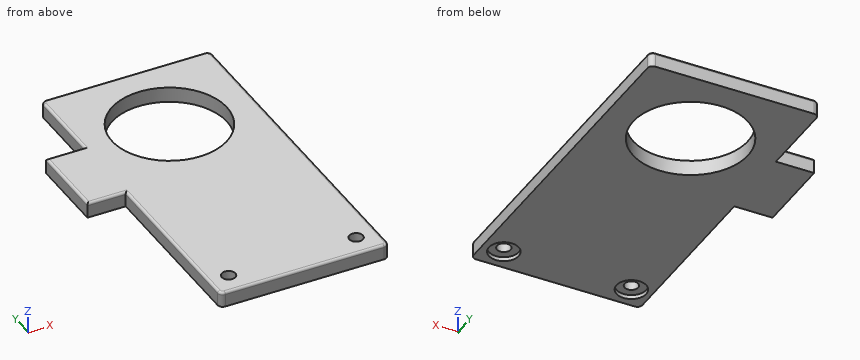
from build123d import *

# Parameters (mm, degrees)
SKETCH_1_R          = 6.75
EXTRUDE_1_DEPTH     = 1.8
SKETCH_2_R          = 0.8
CUT_EXTRUDE_1_DEPTH = 2
SKETCH_3_R          = 1.75
CUT_EXTRUDE_2_DEPTH = 0.5
SKETCH_4_W          = 4.5
SKETCH_4_H          = 9.8
EXTRUDE_2_DEPTH     = 1.8
SKETCH_5_R          = 1.75
EXTRUDE_3_DEPTH     = 1.3
SKETCH_6_R          = 1.75
EXTRUDE_4_DEPTH     = 1.8
EXTRUDE_5_DEPTH     = 1.8
CUT_EXTRUDE_3_DEPTH = 10
FILLET_1_R          = 0.7
CUT_EXTRUDE_4_DEPTH = 10
FILLET_2_R          = 0.3


with BuildPart() as part:
    # 草图1 → 凸台-拉伸1 (new body)
    with BuildSketch(Plane.XY):
        with BuildLine():
            Line((0.7, 0), (19.5, 0))
            ThreePointArc((19.5, 0), (19.994974747, -0.205025253), (20.2, -0.7))
            Line((20.2, -0.7), (20.2, -39.6))
            ThreePointArc((20.2, -39.6), (19.994974747, -40.094974747), (19.5, -40.3))
            Line((19.5, -40.3), (0.7, -40.3))
            ThreePointArc((0.7, -40.3), (0.205025253, -40.094974747), (0, -39.6))
            Line((0, -39.6), (0, -0.7))
            ThreePointArc((0, -0.7), (0.205025253, -0.205025253), (0.7, 0))
        make_face()
        with Locations((10.1, -10.1)):
            Circle(SKETCH_1_R, mode=Mode.SUBTRACT)
    extrude(amount=EXTRUDE_1_DEPTH)

    # 草图2 → 切除-拉伸1 (cut)
    with BuildSketch(Plane.XY.offset(1.8)):
        with Locations((17.6, -2.6)):
            Circle(SKETCH_2_R)
        with Locations((17.6, -37.6)):
            Circle(SKETCH_2_R)
        with Locations((2.6, -37.6)):
            Circle(SKETCH_2_R)
        with Locations((2.6, -2.6)):
            Circle(SKETCH_2_R)
    extrude(amount=-CUT_EXTRUDE_1_DEPTH, mode=Mode.SUBTRACT)

    # 草图3 → 切除-拉伸2 (cut)
    with BuildSketch(Plane(origin=(0, 0, 0), x_dir=(-1, 0, 0), z_dir=(0, 0, -1))):
        with Locations((-17.6, -2.6)):
            Circle(SKETCH_3_R)
        with Locations((-2.6, -2.6)):
            Circle(SKETCH_3_R)
        with Locations((-17.6, -37.6)):
            Circle(SKETCH_3_R)
        with Locations((-2.6, -37.6)):
            Circle(SKETCH_3_R)
    extrude(amount=-CUT_EXTRUDE_2_DEPTH, mode=Mode.SUBTRACT)

    # 草图4 → 凸台-拉伸2 (add)
    with BuildSketch(Plane(origin=(0, 0, 0), x_dir=(-1, 0, 0), z_dir=(0, 0, -1))):
        with Locations((2.25, -14.4)):
            Rectangle(SKETCH_4_W, SKETCH_4_H)
    extrude(amount=-EXTRUDE_2_DEPTH)

    # 草图5 → 凸台-拉伸3 (add)
    with BuildSketch(Plane(origin=(0, 0, 0.5), x_dir=(-1, 0, 0), z_dir=(0, 0, -1))):
        with Locations((-2.6, -2.6)):
            Circle(SKETCH_5_R)
        with Locations((-17.6, -2.6)):
            Circle(SKETCH_5_R)
    extrude(amount=-EXTRUDE_3_DEPTH)

    # 草图6 → 凸台-拉伸4 (add)
    with BuildSketch(Plane(origin=(0, 0, 0), x_dir=(-1, 0, 0), z_dir=(0, 0, -1))):
        with Locations((-17.6, -2.6)):
            Circle(SKETCH_6_R)
        with Locations((-2.6, -2.6)):
            Circle(SKETCH_6_R)
    extrude(amount=-EXTRUDE_4_DEPTH)

    # 草图8 → 凸台-拉伸5 (add)
    with BuildSketch(Plane(origin=(0, 0, 0), x_dir=(-1, 0, 0), z_dir=(0, 0, -1))):
        Polygon((-0.7, 0), (0, 0), (0, -0.7), align=None)
        Polygon((-0.7, -40.3), (0, -40.3), (0, -39.6), align=None)
    extrude(amount=-EXTRUDE_5_DEPTH)

    # 草图9 → 切除-拉伸3 (cut)
    with BuildSketch(Plane(origin=(0, 0, 0), x_dir=(-1, 0, 0), z_dir=(0, 0, -1))):
        Polygon((0, -19.3), (0, -40.3), (-0.15, -40.3), (-0.15, -19.15), (4.35, -19.15), (4.35, -9.65), (-0.15, -9.65), (-0.15, 0), (0, 0), (0, -9.5), (4.5, -9.5), (4.5, -19.3), align=None)
    extrude(amount=-CUT_EXTRUDE_3_DEPTH, mode=Mode.SUBTRACT)

    # 圆角1
    fillet_1_edges = [part.edges().sort_by_distance(p)[0] for p in [
        (0.15, -40.3, 0.9),
        (0.15, 0, 0.9),
    ]]
    fillet(fillet_1_edges, radius=FILLET_1_R)

    # 草图10 → 切除-拉伸4 (cut)
    with BuildSketch(Plane(origin=(0, 0, 0), x_dir=(-1, 0, 0), z_dir=(0, 0, -1))):
        with BuildLine():
            ThreePointArc((-20.2, -39.6), (-19.994974747, -40.094974747), (-19.5, -40.3))
            Line((-19.5, -40.3), (-0.85, -40.3))
            ThreePointArc((-0.85, -40.3), (-0.355025253, -40.094974747), (-0.15, -39.6))
            Line((-0.15, -39.6), (-0.15, -19.15))
            Line((-0.15, -19.15), (4.35, -19.15))
            Line((4.35, -19.15), (4.35, -9.65))
            Line((4.35, -9.65), (-0.15, -9.65))
            Line((-0.15, -9.65), (-0.15, -0.7))
            ThreePointArc((-0.15, -0.7), (-0.355025253, -0.205025253), (-0.85, 0))
            Line((-0.85, 0), (-19.5, 0))
            ThreePointArc((-19.5, 0), (-19.994974747, -0.205025253), (-20.2, -0.7))
            Line((-20.2, -0.7), (-20.2, -39.6))
        make_face()
        with BuildLine():
            ThreePointArc((-20.1, -39.6), (-19.924264069, -40.024264069), (-19.5, -40.2))
            Line((-19.5, -40.2), (-0.85, -40.2))
            ThreePointArc((-0.85, -40.2), (-0.425735931, -40.024264069), (-0.25, -39.6))
            Line((-0.25, -39.6), (-0.25, -19.05))
            Line((-0.25, -19.05), (4.25, -19.05))
            Line((4.25, -19.05), (4.25, -9.75))
            Line((4.25, -9.75), (-0.25, -9.75))
            Line((-0.25, -9.75), (-0.25, -0.7))
            ThreePointArc((-0.25, -0.7), (-0.425735931, -0.275735931), (-0.85, -0.1))
            Line((-0.85, -0.1), (-19.5, -0.1))
            ThreePointArc((-19.5, -0.1), (-19.924264069, -0.275735931), (-20.1, -0.7))
            Line((-20.1, -0.7), (-20.1, -39.6))
        make_face(mode=Mode.SUBTRACT)
    extrude(amount=-CUT_EXTRUDE_4_DEPTH, mode=Mode.SUBTRACT)

    # 圆角2
    fillet_2_edges = [part.edges().sort_by_distance(p)[0] for p in [
        (19.924264069, -40.024264069, 1.8),
        (10.175, -40.2, 1.8),
        (0.425735931, -40.024264069, 1.8),
        (0.25, -29.325, 1.8),
        (-2, -19.05, 1.8),
        (-4.25, -14.4, 1.8),
        (-2, -9.75, 1.8),
        (0.25, -5.225, 1.8),
        (0.425735931, -0.275735931, 1.8),
        (10.175, -0.1, 1.8),
        (19.924264069, -0.275735931, 1.8),
        (20.1, -20.15, 1.8),
    ]]
    fillet(fillet_2_edges, radius=FILLET_2_R)


solid = part.part
Check sheet for the modelled part. Datum: model origin and axes. Units: mm. Coordinates: 2 decimals unless noted, no trailing zeros. Loops run counter-clockwise (first coordinate to the right, second up) from the corner with the lowest first, then second, coordinate; pieces in that order, holes last. Notation, with made-up numbers: (-35.5, 14.25) -> (-1.5, 14.25) arc R31 cw to (-1.5, 40.25) -> close; hole circle Ø4 at (-4.75, -27). An arc over 180 degrees is marked (long way). Answer in a Markdown table with one row per item.
1. Sectioned sample at A-A, the plane x = 10.1. Record the boundary of the cut face in (y, z).
Check values:
| item | result |
|---|---|
| outline | (-40.2, 0) -> (-16.85, 0) -> (-16.85, 1.8) -> (-39.9, 1.8) arc R0.3 ccw to (-40.2, 1.5) -> close; (-3.35, 0) -> (-0.1, 0) -> (-0.1, 1.5) arc R0.3 ccw to (-0.4, 1.8) -> (-3.35, 1.8) -> close |
2. Material ranges on line 1 along X through (y, z) = (-37.6, 0.9); line 2 along Y through (x, z) = (10.1, 1.15); line 3 along Y through (x, z) = (2.6, 0.25), recorded low to high. Write a range as [from, to].
Check values:
| item | result |
|---|---|
| line 1 | x = [0.25, 1.8], [3.4, 16.8], [18.4, 20.1] |
| line 2 | y = [-40.2, -16.85], [-3.35, -0.1] |
| line 3 | y = [-40.2, -39.35], [-35.85, -0.1] |
3. Go/stop test with flat-tipped pins: pin 1 (1 mm diameter, centred on x = 3.5, y = -37.5, fed in from -Z); pin 2 (0.8 mm diameter, centred on x = -3, z = 0.5, fed in from +Y); pin 3 (0.8 mm diameter, centred on y = -33, z = 1, fed in from -X). Record where each tip stops, or that it passes through.
Check values:
| item | result |
|---|---|
| pin 1 | stops at z = 0.5 |
| pin 2 | stops at y = -9.75 |
| pin 3 | stops at x = 0.25 |
4. Sectioned sample at C-C, the plane y = -8. Record the boundary of the cut face in (x, z), then the cut area to 3 significant figures.
Check values:
| item | result |
|---|---|
| outline | (0.25, 0) -> (3.68, 0) -> (3.68, 1.8) -> (0.55, 1.8) arc R0.3 ccw to (0.25, 1.5) -> close; (16.52, 0) -> (20.1, 0) -> (20.1, 1.5) arc R0.3 ccw to (19.8, 1.8) -> (16.52, 1.8) -> close |
| area | 12.6 mm2 |
5. Sectioned sample at D-D, the plane x = 2.6. Record the boundary of the cut face in (y, z).
Check values:
| item | result |
|---|---|
| outline | (-40.2, 0) -> (-39.35, 0) -> (-39.35, 0.5) -> (-38.4, 0.5) -> (-38.4, 1.8) -> (-39.9, 1.8) arc R0.3 ccw to (-40.2, 1.5) -> close; (-36.8, 0.5) -> (-35.85, 0.5) -> (-35.85, 0) -> (-0.1, 0) -> (-0.1, 1.5) arc R0.3 ccw to (-0.4, 1.8) -> (-36.8, 1.8) -> close |
6. Sectioned sample at B-B, the plane z = 1.05. Record the boundary of the cut face in (x, y).
Check values:
| item | result |
|---|---|
| outline | (-4.25, -19.05) -> (0.25, -19.05) -> (0.25, -39.6) arc R0.6 ccw to (0.85, -40.2) -> (19.5, -40.2) arc R0.6 ccw to (20.1, -39.6) -> (20.1, -0.7) arc R0.6 ccw to (19.5, -0.1) -> (0.85, -0.1) arc R0.6 ccw to (0.25, -0.7) -> (0.25, -9.75) -> (-4.25, -9.75) -> close; hole circle Ø1.6 at (2.6, -37.6); hole circle Ø13.5 at (10.1, -10.1); hole circle Ø1.6 at (17.6, -37.6) |
